Source: three-view drawing plus pictorial views. Frame: mm from the lowest corner of the part. A direction names the side the tool comes from. Round coordinates to 2 decimals unless told otherwise and drop trailing zeros. Loops run counter-clockwise (first coordinate to the right, second up) from the corner with the lowest first, then second, coordinate; pieces in that order, holes last. Notation, with made-up numbers: M 23,2 L 38,2 A18 ccw 38,19 Z; hole C -23.5,70.25 d6. An arc over 180 degrees is marked long. Write each question's results on one line, items separated by ' | '.
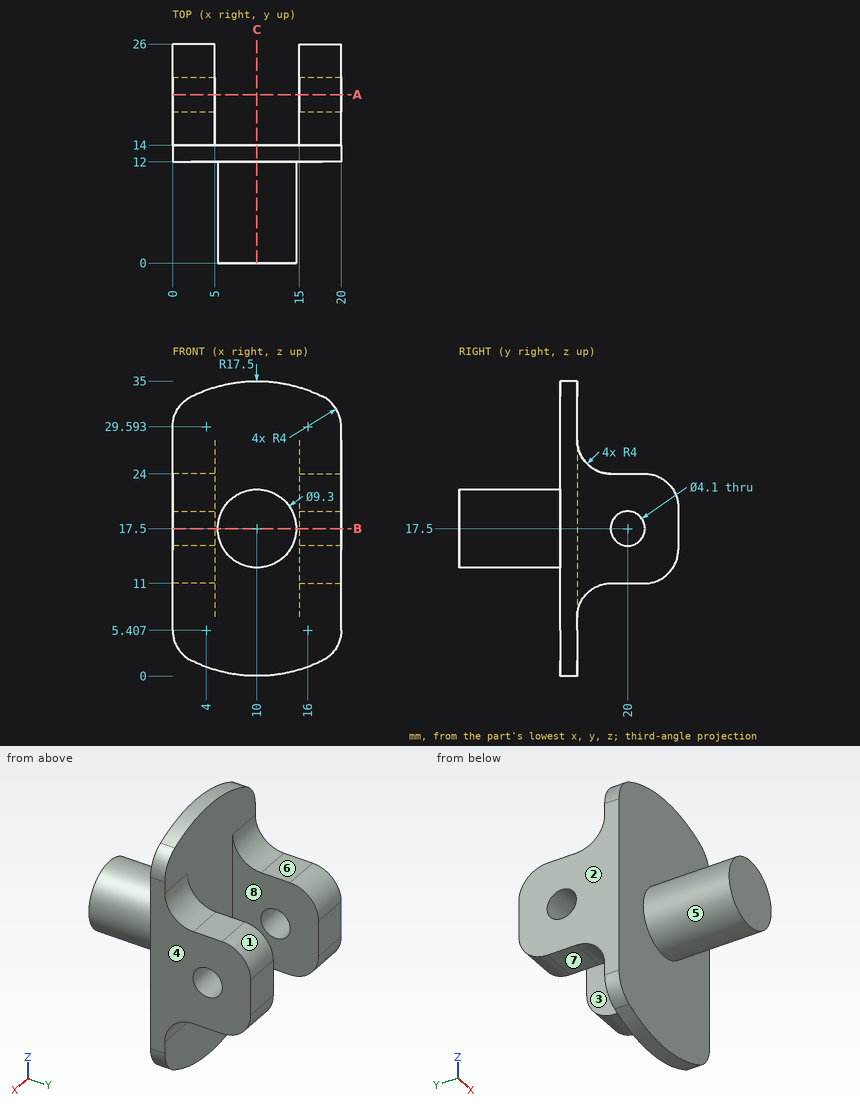
1. Access query for the marked faces 5, 6, 7 and 8. Directions: +Z, -Z, +X, -X, +Y, -Y. A direction counts if a zero-diameter tool reaches every point of the face in a straight line with its end or side. Return the directions, or none.
Answer key:
face 5: -Y | face 6: +Z, +X, -X, +Y | face 7: -Z, +X, -X, +Y | face 8: +Z, -Z, +Y
2. Section B-B (z = 17.5). Output: boundary loops of the cut face in (x, y).
Answer key:
outline: M 0,12 L 5.35,12 L 5.35,0 L 14.65,0 L 14.65,12 L 20,12 L 20,17.95 L 15,17.95 L 15,14 L 5,14 L 5,17.95 L 0,17.95 Z; M 0,22.05 L 5,22.05 L 5,26 L 0,26 Z; M 15,22.05 L 20,22.05 L 20,26 L 15,26 Z
3. Draft query along X for the marked faces 1, 2, 3 and 4. Return one class per face: pulls with the +X half, pulls with the -X half, needs draft (parallel to the pull), parting line crosses it, or undercut.
Answer key:
face 1: needs draft | face 2: pulls with the -X half | face 3: undercut | face 4: pulls with the +X half
4. Section A-A (y = 20). Output: boundary loops of the cut face in (x, z).
Answer key:
outline: M 0,11 L 5,11 L 5,15.45 L 0,15.45 Z; M 0,19.55 L 5,19.55 L 5,24 L 0,24 Z; M 15,11 L 20,11 L 20,15.45 L 15,15.45 Z; M 15,19.55 L 20,19.55 L 20,24 L 15,24 Z
5. Ray query, probe 1 along Y at (x, z) = (1.2, 17.5); probe 2 along X at (y, z) = (16, 12.5); probe 3 along Y at (x, z) = (12.25, 23.5). Return the intervals inside material, ascending.
Answer key:
probe 1: y = 12 to 17.95, 22.05 to 26 | probe 2: x = 0 to 5, 15 to 20 | probe 3: y = 12 to 14
6. Pin query (flat end, axial travel): P1, Ø2, axis at x = 12.5, z = 12.5, coming from the +Y side; P2, Ø2, axis at x = 3.5, y = 20.5, coming from the +Z side; P3, Ø4.5, axis at x = 18.5, y = 19.5, coming from the -Z side; P4, Ø3, axis at y = 22, z = 8.5, coming from the +X side. Return the tip coordinate at first contact, or that it passes through.
Answer key:
P1: stops at y = 14 | P2: stops at z = 24 | P3: stops at z = 10.93 | P4: passes through
7. Section C-C (x = 10). Output: boundary loops of the cut face in (y, z).
Answer key:
outline: M 0,12.85 L 12,12.85 L 12,0 L 14,0 L 14,35 L 12,35 L 12,22.15 L 0,22.15 Z
